from build123d import *

# Parameters (mm, degrees)
SKETCH_1_R               = 2.5
EXTRUDE_1_DEPTH          = 5
SKETCH_2_R               = 2.5
CUT_EXTRUDE_1_DEPTH      = 20
PATTERN_CIRCULAR_1_COUNT = 6


with BuildPart() as part:
    # Эскиз1 → Бобышка-Вытянуть1 (new body)
    with BuildSketch(Plane(origin=(0, 0, 0), x_dir=(1, 0, 0), z_dir=(0, 1, 0))):
        with BuildLine():
            Line((45.954799299, 14.53947803), (47.297271453, -9.284832422))
            ThreePointArc((47.297271453, -9.284832422), (2.711712187, -48.123659639), (-45.954799299, -14.53947803))
            Line((-45.954799299, -14.53947803), (-47.297271453, 9.284832422))
            ThreePointArc((-47.297271453, 9.284832422), (-2.711712187, 48.123659639), (45.954799299, 14.53947803))
        make_face()
        with Locations(Location((0, 0, 0), (0, 0, 270))):
            Circle(SKETCH_1_R, mode=Mode.SUBTRACT)
    extrude(amount=EXTRUDE_1_DEPTH)

    # Эскиз2 → Вырез-Вытянуть1 (cut)
    with BuildSketch(Plane(origin=(0, 5, 0), x_dir=(1, 0, 0), z_dir=(0, 1, 0))):
        with Locations(Location((0, 39.1, 0), (0, 0, 270))):
            Circle(SKETCH_2_R)
    cut_extrude_1 = extrude(amount=-CUT_EXTRUDE_1_DEPTH, mode=Mode.SUBTRACT)

    # Круговой массив1: Вырез-Вытянуть1 ×6 about axis
    pattern_circular_1_axis = Axis((0, 0, 0), (0, 1, 0))
    for i in range(1, PATTERN_CIRCULAR_1_COUNT):
        add(cut_extrude_1.rotate(pattern_circular_1_axis, i * 360 / PATTERN_CIRCULAR_1_COUNT), mode=Mode.SUBTRACT)


solid = part.part
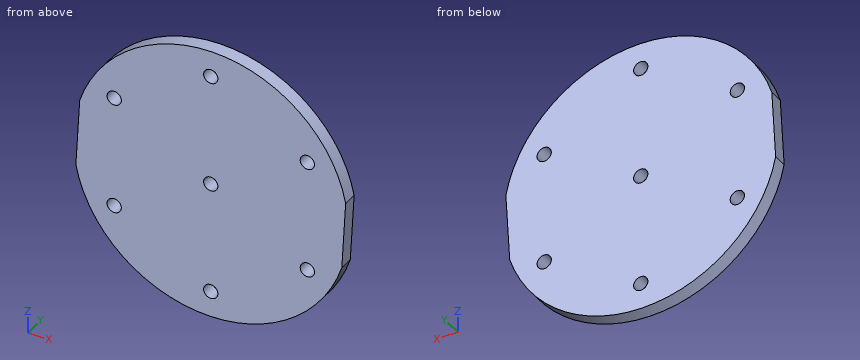
CAD build for the part. Positions are in the model's coordinates, mm. Give positions to 0.01 mm unless a question says otherwise; leave off trailing zeros. Loops run counter-clockwise (first coordinate to the right, second up) from the corner with the lowest first, then second, coordinate; pieces in that order, holes last. Notation, with made-up numbers: M -36.5,0.5 L -3.5,0.5 A16 ccw -3.5,18.5 Z; hole C 16,62 d11. An arc over 180 degrees is marked long. Answer in a Markdown table with one row per item. Add a question column.
Item 1: Probe probe 1 along Z at (x, y) = (-1, 0.4); probe 2 along X at (y, z) = (1.95, 19.55); probe 3 along X at (y, z) = (3.7, 1.5). List the from-to ranges inside material, lowest first.
Item 2: Band-saw the part on A-A on x = 0. Give the cut face in (y, z).
Item 3: Band-saw the part on D-D on y = 2.15. Give the cut face in (x, z).
Item 4: Drop flat-ended pins along their axis: P1, Ø8, axis at x = 0, z = 39.1, coming from the -Y side; P2, Ø1, axis at x = -27.5, y = 0.5, coming from the -Z side; P3, Ø3, axis at y = 3, z = 4, coming from the +X side. Give the stop position or say it passes through.
Item 5: Band-saw the part on C-C on z = 0. Give the cut face in (x, y).
Item 6: Band-saw the part on B-B on z = 19.55. Give the cut face in (x, y), then the cut area to 3 significant figures.
Reply:
| question | item | result |
|---|---|---|
| 1 | probe 1 | z = -48.19 to -41.39, -36.81 to -2.29, 2.29 to 36.81, 41.39 to 48.19 |
| 1 | probe 2 | x = -44.06 to -36.36, -31.36 to 31.36, 36.36 to 44.06 |
| 1 | probe 3 | x = -46.69 to -2, 2 to 46.86 |
| 2 | outline | M 0,-48.2 L 5,-48.2 L 5,-41.6 L 0,-41.6 Z; M 0,-36.6 L 5,-36.6 L 5,-2.5 L 0,-2.5 Z; M 0,2.5 L 5,2.5 L 5,36.6 L 0,36.6 Z; M 0,41.6 L 5,41.6 L 5,48.2 L 0,48.2 Z |
| 3 | outline | M -47.3,-9.28 A48.2 ccw 45.95,-14.54 L 47.3,9.28 A48.2 ccw -45.95,14.54 Z; hole C -33.86,-19.55 d5; hole C -33.86,19.55 d5; hole C 0,-39.1 d5; hole C 0,0 d5; hole C 0,39.1 d5; hole C 33.86,-19.55 d5; hole C 33.86,19.55 d5 |
| 4 | P1 | stops at y = 0 |
| 4 | P2 | stops at z = -39.93 |
| 4 | P3 | stops at x = 47.08 |
| 5 | outline | M -46.77,0 L -2.5,0 L -2.5,5 L -46.77,5 Z; M 2.5,0 L 46.77,0 L 46.77,5 L 2.5,5 Z |
| 6 | outline | M -44.06,0 L -36.36,0 L -36.36,5 L -44.06,5 Z; M -31.36,0 L 31.36,0 L 31.36,5 L -31.36,5 Z; M 36.36,0 L 44.06,0 L 44.06,5 L 36.36,5 Z |
| 6 | area | 391 mm^2 |
